```python
from build123d import *

# Parameters (mm, degrees)
PAD002_DEPTH = 0.8
SKETCH079_R  = 2.7
PAD003_DEPTH = 5
FILLET001_R  = 0.4


with BuildPart() as part:
    # Sketch078 → Pad002 (new body)
    with BuildSketch(Plane.XZ):
        with BuildLine():
            ThreePointArc((2.7, 5.5), (0, 8.2), (-2.7, 5.5))
            Line((-2.7, 5.5), (-2.7, -5.500015))
            ThreePointArc((-2.7, -5.500015), (0, -8.2), (2.7, -5.500015))
            Line((2.7, 5.5), (2.7, -5.500015))
        make_face()
    extrude(amount=PAD002_DEPTH)

    # Sketch079 → Pad003 (join)
    with BuildSketch(Plane.XZ):
        with Locations((0, 5.5)):
            Circle(SKETCH079_R)
        with Locations((0, -5.5)):
            Circle(SKETCH079_R)
    extrude(amount=PAD003_DEPTH)

    # Fillet001
    fillet001_edges = [part.edges().sort_by_distance(p)[0] for p in [
        (-2.7, -5, -5.5),
        (-2.7, -5, 5.5),
    ]]
    fillet(fillet001_edges, radius=FILLET001_R)


solid = part.part
```
Source: CAD feature listing. Evaluate the final solid. Frame: model axes, mm. Coordinates: 2 decimals unless noted, no trailing zeros. Write each loop counter-clockwise with the first axis right and the second up, starting at its lowest first coordinate (ties: lowest second). Pieces come first, ordered by that corner, then holes. Notation, with made-up numbers: (84, -32) - (116, -32) arc R31 ccw to (116, 2) - close; hole circle Ø10 at (59.25, -27.75). An arc over 180 degrees is marked (long way). Answer as a JSON object with one key per item and string values.
Q1. Section query D-D, the plane y = -0.6. Output: boundary loops of the cut face in (x, z), plus the area to 3 significant figures.
Ans:
{"outline": "(-2.7, -5.5) arc R2.7 ccw to (2.7, -5.5) - (2.7, 5.5) arc R2.7 ccw to (-2.7, 5.5) - close", "area": "82.3 mm2"}
Q2. Draft query along Z for faces 1 (the flat face through (0, -0.8, 0)), 2 (the flat face through (0, -5, 6)), 3 (the cylindrical face through (-0.351, -2.268, 8.177)). Return one class per face: released by +Z, released by -Z, zero draft, split by the parting line, or undercut.
Ans:
{"face 1": "undercut", "face 2": "zero draft", "face 3": "undercut"}
Q3. Section query A-A, the plane x = 0. Output: boundary loops of the cut face in (y, z).
Ans:
{"outline": "(-5, -7.8) arc R0.4 ccw to (-4.6, -8.2) - (0, -8.2) - (0, 8.2) - (-4.6, 8.2) arc R0.4 ccw to (-5, 7.8) - (-5, 3.2) arc R0.4 ccw to (-4.6, 2.8) - (-0.8, 2.8) - (-0.8, -2.8) - (-4.6, -2.8) arc R0.4 ccw to (-5, -3.2) - close"}
Q4. Material intervals for line 1 (Y direction, x = 1.9, z = 1); line 2 (Z direction, x = 1.15, y = -2.15); line 3 (Z direction, x = 2.25, y = -2.95), sorted ascending. Write a range as [from, to].
Ans:
{"line 1": "y = [-0.8, 0]", "line 2": "z = [-7.94, -3.06], [3.06, 7.94]", "line 3": "z = [-6.99, -4.01], [4.01, 6.99]"}
Q5. Section query B-B, the plane y = -3.55. Output: boundary loops of the cut face in (x, z).
Ans:
{"outline": "circle Ø5.4 at (0, -5.5); circle Ø5.4 at (0, 5.5)"}
Q6. First-contact query: pin 1 Ø1 at (y, z) = (-2, -0.5) entering from -X; pin 2 Ø3 at (x, z) = (1.5, -0.5) entering from -Y; pin 3 Ø1.5 at (x, y) = (-1.5, -3.5) entering from +Z. Flat tips, straight axial feed; report the tip coordinate or a pass-through.
Ans:
{"pin 1": "passes through", "pin 2": "stops at y = -0.8", "pin 3": "stops at z = 8.09"}
Q7. Section query C-C, the plane z = -1.75. Output: boundary loops of the cut face in (x, y).
Ans:
{"outline": "(-2.7, -0.8) - (2.7, -0.8) - (2.7, 0) - (-2.7, 0) - close"}
